Check sheet for the modelled part. Datum: model origin and axes. Units: mm. Face numbers are marked on the shaded views. A direction names the side the tool comes from. Round coordinates to 2 decimals unless told otherwise and drop trailing zeros. Loops run counter-clockwise (first coordinate to the right, second up) from the corner with the lowest first, then second, coordinate; pieces in that order, holes last. Notation, with made-up numbers: (35, 44) -> (44, 44) arc R24 cw to (44, 80) -> close; hole circle Ø7 at (24, -10.5). An arc over 180 degrees is marked (long way). One line per question, with ' | ' between items.
```python
from build123d import *

# Parameters (mm, degrees)
F1_DEPTH = 130
F3_D     = 7
F5_D     = 5
F7_DEPTH = 25


# Not quite as in the source:
# - a feature names something its author has since deleted; it is built from what else it names


with BuildPart() as f1:
    # F0 (on Front) → F1 (new body, symmetric)
    with BuildSketch(Plane.XZ):
        Polygon((0, 30), (0, 0), (3, 0), (3, 27), (30, 27), (30, 30), align=None)
    extrude(amount=F1_DEPTH, both=True)

    # F3 (through all)
    with Locations(Plane(origin=(0, 0, 0), x_dir=(0, -1, 0), z_dir=(-1, 0, 0))):
        with Locations((-115, 10), (-30, 10), (30, 10), (115, 10)):
            Hole(F3_D / 2)

    # F5 (through all)
    with Locations(Plane.XY.offset(30)):
        with Locations((14.7187495604, -120), (14.7187495604, -80), (14.7187495604, 0), (14.7187495604, 80), (14.7187495604, 120)):
            Hole(F5_D / 2)

    # F6 (on face) → F7 (cut)
    with BuildSketch(Plane.YZ.offset(3)):
        Polygon((-130, 15), (-130, 0), (-115, 0), align=None)
        Polygon((130, 15), (115, 0), (130, 0), align=None)
    extrude(amount=-F7_DEPTH, mode=Mode.SUBTRACT)


solid = f1.part
```
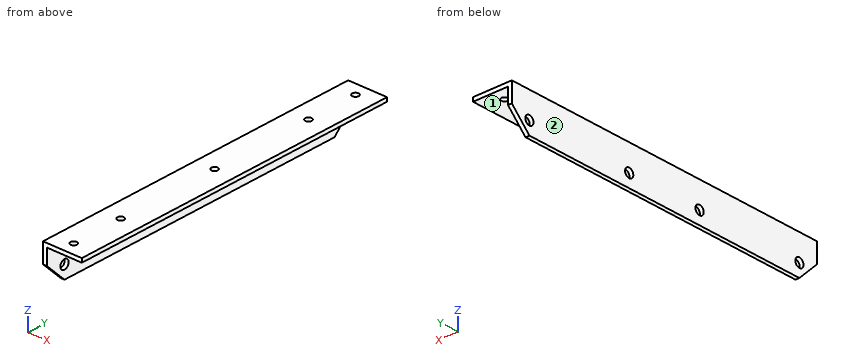
(1) Sectioned sample at C-C, the plane x = 26.5. Record the cut outline in (y, z).
Answer:
outline: (-130, 27) -> (130, 27) -> (130, 30) -> (-130, 30) -> close
(2) Set-up check for the marked faces 1 and 2: record each of +Z, -Z, +X, -X, +Y, -Y from which the full face is reachable in a straight line by a thin tool's end or side.
Answer:
face 1: -Z, +X, +Y, -Y | face 2: +Z, -Z, -X, +Y, -Y
(3) Scan lines: probe 1 along Z at (x, y) = (2.15, 30); probe 2 along X at (y, z) = (-87, 21); probe 3 along Z at (x, y) = (6, -107). Record each from-to range of solid material in increasing order.
Answer:
probe 1: z = 0 to 6.5, 13.5 to 30 | probe 2: x = 0 to 3 | probe 3: z = 27 to 30
(4) Sectioned sample at A-A, the plane y = -80. Record the cut outline in (x, z), and give its area (3 significant figures).
Answer:
outline: (0, 0) -> (3, 0) -> (3, 27) -> (12.22, 27) -> (12.22, 30) -> (0, 30) -> close; (17.22, 27) -> (30, 27) -> (30, 30) -> (17.22, 30) -> close | area: 156 mm2
(5) Sectioned sample at D-D, the plane z = 17.75. Record the cut outline in (x, y), and give its area (3 significant figures).
Answer:
outline: (0, -130) -> (3, -130) -> (3, 130) -> (0, 130) -> close | area: 780 mm2
(6) Go/stop test with flat-tipped pins: pin 1 (4.5 mm diameter, centred on x = 14.72, y = -120, fed in from -Z); pin 2 (11 mm diameter, centred on y = -30, z = 10, fed in from +X); pin 3 (5 mm diameter, centred on x = 26, y = -81.5, fed in from -Z). Record where each tip stops, or that it passes through.
Answer:
pin 1: passes through | pin 2: stops at x = 3 | pin 3: stops at z = 27
(7) Sectioned sample at B-B, the plane y = 30. Record the cut outline in (x, z).
Answer:
outline: (0, 0) -> (3, 0) -> (3, 6.5) -> (0, 6.5) -> close; (0, 13.5) -> (3, 13.5) -> (3, 27) -> (30, 27) -> (30, 30) -> (0, 30) -> close
